```python
from build123d import *

# Parameters (mm, degrees)
SKETCH_1_W          = 416
SKETCH_1_H          = 28
EXTRUDE_677_DEPTH   = 16
FILLET_1_R          = 0.8
CUT_EXTRUDE_1_DEPTH = 417.542914956
CHAMFER_1_SIZE      = 2
HOLE_WIZARD_M10_1_D = 8.5


with BuildPart() as part:
    # 草图1 → Extrude 677 (new body)
    with BuildSketch(Plane.XY):
        Rectangle(SKETCH_1_W, SKETCH_1_H)
    extrude(amount=EXTRUDE_677_DEPTH)

    # 圆角1
    fillet_1_edges = [part.edges().sort_by_distance(p)[0] for p in [
        (0, -14, 16),
        (0, -14, 0),
        (0, 14, 0),
        (0, 14, 16),
    ]]
    fillet(fillet_1_edges, radius=FILLET_1_R)

    # 草图2 → 切除-拉伸1 (cut, through all)
    with BuildSketch(Plane.ZY.offset(208)):
        with BuildLine():
            Line((16, 13), (0, 13))
            Line((0, 13), (0, 13.2))
            ThreePointArc((0, 13.2), (0.234314575, 13.765685425), (0.8, 14))
            Line((0.8, 14), (15.2, 14))
            ThreePointArc((15.2, 14), (15.765685425, 13.765685425), (16, 13.2))
            Line((16, 13.2), (16, 13))
        make_face()
        with BuildLine():
            Line((16, -13), (0, -13))
            Line((0, -13), (0, -13.2))
            ThreePointArc((0, -13.2), (0.234314575, -13.765685425), (0.8, -14))
            Line((0.8, -14), (15.2, -14))
            ThreePointArc((15.2, -14), (15.765685425, -13.765685425), (16, -13.2))
            Line((16, -13.2), (16, -13))
        make_face()
    extrude(amount=-CUT_EXTRUDE_1_DEPTH, mode=Mode.SUBTRACT)

    # 倒角1
    chamfer_1_edges = [part.edges().sort_by_distance(p)[0] for p in [
        (0, 13, 16),
        (0, 13, 0),
        (0, -13, 16),
        (0, -13, 0),
    ]]
    chamfer(chamfer_1_edges, length=CHAMFER_1_SIZE)

    # M10 螺纹孔1 (through all)
    with Locations(Plane.XY.offset(16)):
        with Locations((-147, 0), (-42, 0), (63, 0), (168, 0)):
            Hole(HOLE_WIZARD_M10_1_D / 2)


solid = part.part
```
Design review of the part built by this model. Coordinates are the model's own, in mm. Coordinates: 2 decimals unless noted, no trailing zeros. Order: outer loops, then holes, each group sorted by start corner. A loop starts at its lowest first (then second) coordinate and runs counter-clockwise, first axis right, second up. Notation, with made-up numbers: M -20,-25 L -13,-25 A15 cw -13,-9 Z; hole C -40,-24.75 d3. An arc over 180 degrees is marked long. Answer as a JSON object with one key per item and string values. Group by question number.
1) Wall thickness on L1, parallel to X at y = -0.25, z = 4.5; L2, parallel to Y at x = 63, z = 6; L3, parallel to Y at x = -44, z = 0.5: over which ranges is each line inside the solid? List them lowest first.
2) Mouldability with a two-part tool opening along Y and no side actions: class faces 1 (the flat face through (-208, 0, 8)), 2 (the flat face through (-3, 13, 8)), 3 (the cylindrical face through (172.246, 0.187, 7.888)) as pulls with the +Y half, pulls with the -Y half, needs draft (parallel to the pull), parting line crosses it, or undercut.
3) Add section B-B, the plane x = 82.5. Write out the cut boundary in (y, z), then the cut area to 3 significant figures.
4) Add section A-A, the plane x = -147. Write out the cut boundary in (y, z), then the cut area to 3 significant figures.
Computed values:
{
 "1": {"L1": "x = -208 to -151.24, -142.76 to -46.24, -37.76 to 58.76, 67.24 to 163.76, 172.24 to 208", "L2": "y = -13 to -4.25, 4.25 to 13", "L3": "y = -11.5 to -3.75, 3.75 to 11.5"},
 "2": {"face 1": "needs draft", "face 2": "pulls with the +Y half", "face 3": "undercut"},
 "3": {"outline": "M -13,2 L -11,0 L 11,0 L 13,2 L 13,14 L 11,16 L -11,16 L -13,14 Z", "area": "408 mm^2"},
 "4": {"outline": "M -13,2 L -11,0 L -4.25,0 L -4.25,16 L -11,16 L -13,14 Z; M 4.25,0 L 11,0 L 13,2 L 13,14 L 11,16 L 4.25,16 Z", "area": "272 mm^2"}
}
